Part model, mm, in its own coordinate system. A direction names the side the tool comes from. Give positions to 0.01 mm unless a question says otherwise; leave off trailing zeros. Order: outer loops, then holes, each group sorted by start corner. A loop starts at its lowest first (then second) coordinate and runs counter-clockwise, first axis right, second up. Notation, with made-up numbers: (16.25, 43.5) - (48.25, 43.5) arc R28 ccw to (48.25, 70.5) - close; hole circle Ø9 at (53.5, 26.5). An arc over 180 degrees is marked (long way). One line per item, written item: value.
```python
from build123d import *

# Parameters (mm, degrees)
F1_DEPTH = 50
F2_R     = 7
F3_DEPTH = 16


with BuildPart() as f1:
    # F0 (on Front) → F1 (new body)
    with BuildSketch(Plane.XZ):
        with BuildLine():
            Line((-35, 22), (-35, 0))
            Line((-35, 0), (-23, 0))
            ThreePointArc((-23, 0), (0, 23), (23, 0))
            Line((23, 0), (35, 0))
            Line((35, 0), (35, 22))
            Line((35, 22), (66, 22))
            Line((66, 22), (66, 38))
            Line((66, 38), (-66, 38))
            Line((-66, 38), (-66, 22))
            Line((-66, 22), (-35, 22))
        make_face()
    extrude(amount=F1_DEPTH)

    # F2 (on face) → F3 (cut)
    with BuildSketch(Plane.XY.offset(38)):
        with Locations((49.832433, -25)):
            Circle(F2_R)
        with Locations((-50.167567, -25)):
            Circle(F2_R)
    extrude(amount=-F3_DEPTH, mode=Mode.SUBTRACT)


solid = f1.part
```
1) Slice it at C-C on x = 49. Write the cut outline in (y, z).
Answer:
outline: (-50, 22) - (-31.95, 22) - (-31.95, 38) - (-50, 38) - close; (-18.05, 22) - (0, 22) - (0, 38) - (-18.05, 38) - close
2) Wall check: line 1 along Z through (x, y) = (-60, -2); line 2 along X through (y, z) = (-38.5, 18); line 3 along X through (y, z) = (-26.5, 29). Give the ranges that are in metal, low to high. Write a range as [from, to].
Answer:
line 1: z = [22, 38]
line 2: x = [-35, -14.32], [14.32, 35]
line 3: x = [-66, -57], [-43.33, 43], [56.67, 66]
3) Drop flat-ended pins along their axis: P1, Ø18, axis at x = 49.83, y = -25, coming from the -Z side; P2, Ø1.5, axis at x = 15, y = -23.5, coming from the -Z side; P3, Ø6, axis at y = -8, z = 5, coming from the -X side; P4, Ø12.5, axis at x = -50.17, y = -25, coming from the -Z side. Give the stop position or say it passes through.
Answer:
P1: stops at z = 22
P2: stops at z = 16.76
P3: stops at x = -35
P4: passes through
4) Slice it at B-B on z = 15. Write the cut outline in (x, y).
Answer:
outline: (-35, -50) - (-17.44, -50) - (-17.44, 0) - (-35, 0) - close; (17.44, -50) - (35, -50) - (35, 0) - (17.44, 0) - close
5) Which spindle directions (+Z, -Z, +X, -X, +Y, -Y) get a long thin tool onto all of the face, cutting with end or side? Do faces 1 (the face through (54, -19, 22)), 2 (the face through (29, -25, 0)), 3 (the face through (-58, -25, 22)). Say none if no direction does.
Answer:
face 1: -Z, +X, +Y, -Y
face 2: -Z, +X, -X, +Y, -Y
face 3: -Z, -X, +Y, -Y
6) Two-plate mould, pull along Y, no slides. Class faces 4 (the face through (-29, -25, 0)), 5 (the face through (-0.9, 0, 23.5)), 6 (the face through (-0.9, -50, 23.5)), 7 (the face through (56.3, -27.68, 30.11)): pulls with the +Y half, pulls with the -Y half, needs draft (parallel to the pull), parting line crosses it, or undercut.
Answer:
face 4: needs draft
face 5: pulls with the +Y half
face 6: pulls with the -Y half
face 7: undercut
7) Slice it at D-D on z = 27. Write the cut outline in (x, y), then the cut area to 3 significant figures.
Answer:
outline: (-66, -50) - (66, -50) - (66, 0) - (-66, 0) - close; hole circle Ø14 at (-50.17, -25); hole circle Ø14 at (49.83, -25)
area: 6,290 mm2
8) Slice it at A-A on y = -47. Write the cut outline in (x, z).
Answer:
outline: (-66, 22) - (-35, 22) - (-35, 0) - (-23, 0) arc R23 cw to (23, 0) - (35, 0) - (35, 22) - (66, 22) - (66, 38) - (-66, 38) - close
